Read the model definition and answer for the solid it produces. Units are mm, in the model's axes. Face numbers are marked on the shaded views. Coordinates: 2 decimals unless noted, no trailing zeros. Write each loop counter-clockwise with the first axis right and the second up, starting at its lowest first coordinate (ties: lowest second). Pieces come first, ordered by that corner, then holes. Notation, with made-up numbers: M 26.25,-16 L 78.25,-16 A16 cw 78.25,12 Z; hole C -22.75,-36 d4. An arc over 180 degrees is marked long. Write item = value, one per line.
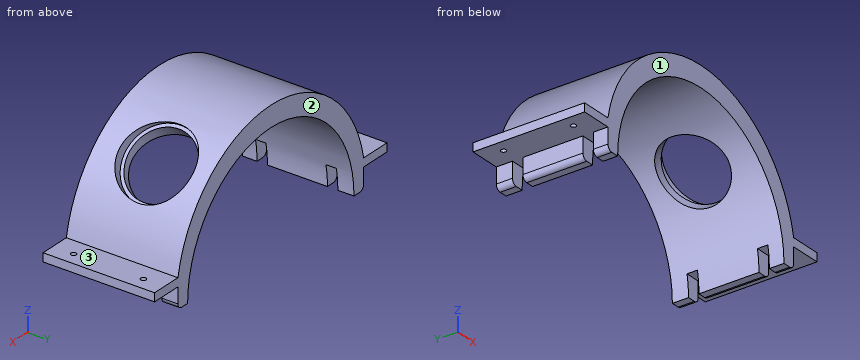
from build123d import *

# Parameters (mm, degrees)
BOSS_EXTRUDE1_DEPTH = 107
SKETCH2_R           = 2.5
CUT_EXTRUDE1_DEPTH  = 336.0337743
SKETCH3_R           = 35
CUT_EXTRUDE2_DEPTH  = 10
SKETCH4_R           = 31.778321021
CUT_EXTRUDE3_DEPTH  = 25
CUT_EXTRUDE4_REACH  = 337.034
SKETCH5_W           = 15.542799326
SKETCH5_H           = 10
SKETCH5_W_2         = 18.63674205


with BuildPart() as part:
    # Sketch1 → Boss-Extrude1 (new body)
    with BuildSketch(Plane(origin=(0, 0, 0), x_dir=(1, 0, 0), z_dir=(0, 1, 0))):
        with BuildLine():
            Line((0, 0), (0, -8))
            Line((0, -8), (30, -8))
            ThreePointArc((30, -8), (149.5, -106.759683035), (269, -8))
            Line((269, -8), (299, -8))
            Line((299, -8), (299, 0))
            Line((299, 0), (269, 0))
            Line((269, 0), (269, 15))
            ThreePointArc((269, 15), (267.535533906, 18.535533906), (264, 20))
            Line((264, 20), (256.5, 20))
            ThreePointArc((256.5, 20), (149.5, -87.000008561), (42.5, 20))
            Line((42.5, 20), (35, 20))
            ThreePointArc((35, 20), (31.464466094, 18.535533906), (30, 15))
            Line((30, 15), (30, 0))
            Line((30, 0), (0, 0))
        make_face()
    extrude(amount=BOSS_EXTRUDE1_DEPTH)

    # Sketch2 → Cut-Extrude1 (cut, through all)
    with BuildSketch(Plane(origin=(0, 0, 0), x_dir=(-1, 0, 0), z_dir=(0, 0, -1))):
        with Locations((-286.5, 87)):
            Circle(SKETCH2_R)
        with Locations((-286.5, 20)):
            Circle(SKETCH2_R)
        with Locations((-12.5, 87)):
            Circle(SKETCH2_R)
        with Locations((-12.5, 20)):
            Circle(SKETCH2_R)
    extrude(amount=-CUT_EXTRUDE1_DEPTH, mode=Mode.SUBTRACT)

    # Sketch3 → Cut-Extrude2 (cut)
    with BuildSketch(Plane(origin=(152.698962186, 0, 153.519285181), x_dir=(0.7089984938103423, 0, -0.7052099940972661), z_dir=(0.7052099940972661, 0, 0.7089984938103423))):
        with Locations((109.109605527, 56.865799068)):
            Circle(SKETCH3_R)
    extrude(amount=-CUT_EXTRUDE2_DEPTH, mode=Mode.SUBTRACT)

    # Sketch4 → Cut-Extrude3 (cut)
    with BuildSketch(Plane(origin=(145.646862245, 0, 146.429300243), x_dir=(0.7089984938103423, 0, -0.7052099940972661), z_dir=(0.7052099940972661, 0, 0.7089984938103423))):
        with Locations((109.109605527, 56.865799068)):
            Circle(SKETCH4_R)
    extrude(amount=-CUT_EXTRUDE3_DEPTH, mode=Mode.SUBTRACT)

    # Cut-Extrude4: up to this face of the body (flat: up to its plane)
    cut_extrude4_end = Plane(part.part.faces().sort_by_distance((260.25, 53.5, -20))[0])
    # Sketch5 → Cut-Extrude4 (cut, up to the picked face)
    with BuildSketch(Plane(origin=(0, 0, 0), x_dir=(-1, 0, 0), z_dir=(0, 0, -1)), mode=Mode.PRIVATE) as cut_extrude4_sk1:
        with Locations((-261.228600337, 86.535453814)):
            Rectangle(SKETCH5_W, SKETCH5_H)
    cut_extrude4_tool1 = split(extrude(cut_extrude4_sk1.sketch, amount=CUT_EXTRUDE4_REACH, mode=Mode.PRIVATE), bisect_by=cut_extrude4_end, keep=Keep.BOTH, mode=Mode.PRIVATE)
    # Sketch5 → Cut-Extrude4 (cut, up to the picked face)
    with BuildSketch(Plane(origin=(0, 0, 0), x_dir=(-1, 0, 0), z_dir=(0, 0, -1)), mode=Mode.PRIVATE) as cut_extrude4_sk2:
        with Locations((-259.681628975, 19.008712967)):
            Rectangle(SKETCH5_W_2, SKETCH5_H)
    cut_extrude4_tool2 = split(extrude(cut_extrude4_sk2.sketch, amount=CUT_EXTRUDE4_REACH, mode=Mode.PRIVATE), bisect_by=cut_extrude4_end, keep=Keep.BOTH, mode=Mode.PRIVATE)
    # Sketch5 → Cut-Extrude4 (cut, up to the picked face)
    with BuildSketch(Plane(origin=(0, 0, 0), x_dir=(-1, 0, 0), z_dir=(0, 0, -1)), mode=Mode.PRIVATE) as cut_extrude4_sk3:
        with Locations((-39.318371025, 19.008712967)):
            Rectangle(SKETCH5_W_2, SKETCH5_H)
    cut_extrude4_tool3 = split(extrude(cut_extrude4_sk3.sketch, amount=CUT_EXTRUDE4_REACH, mode=Mode.PRIVATE), bisect_by=cut_extrude4_end, keep=Keep.BOTH, mode=Mode.PRIVATE)
    # Sketch5 → Cut-Extrude4 (cut, up to the picked face)
    with BuildSketch(Plane(origin=(0, 0, 0), x_dir=(-1, 0, 0), z_dir=(0, 0, -1)), mode=Mode.PRIVATE) as cut_extrude4_sk4:
        with Locations((-37.771399663, 86.535453814)):
            Rectangle(SKETCH5_W, SKETCH5_H)
    cut_extrude4_tool4 = split(extrude(cut_extrude4_sk4.sketch, amount=CUT_EXTRUDE4_REACH, mode=Mode.PRIVATE), bisect_by=cut_extrude4_end, keep=Keep.BOTH, mode=Mode.PRIVATE)
    add(cut_extrude4_tool1.solids().sort_by(Axis((261.2286, 86.535454, 0), (0, 0, -1)))[0], mode=Mode.SUBTRACT)
    add(cut_extrude4_tool2.solids().sort_by(Axis((259.681629, 19.008713, 0), (0, 0, -1)))[0], mode=Mode.SUBTRACT)
    add(cut_extrude4_tool3.solids().sort_by(Axis((39.318371, 19.008713, 0), (0, 0, -1)))[0], mode=Mode.SUBTRACT)
    add(cut_extrude4_tool4.solids().sort_by(Axis((37.7714, 86.535454, 0), (0, 0, -1)))[0], mode=Mode.SUBTRACT)


solid = part.part
Item 1: Consider line 1 along Y through (x, z) = (286.5, 2); line 2 along Y through (x, z) = (12, 4); line 3 along Z through (x, y) = (12.5, 30). Determine where each line is inside the solid, lowest interval first. Write a range as from..to.
Worked answers:
line_1 = 0..17.5, 22.5..84.5, 89.5..107
line_2 = 0..17.55, 22.45..84.55, 89.45..107
line_3 = 0..8
Item 2: Find section D-D (x = 149.5). Determine the outline of the cut face in (y, z), and give its area (3 significant figures).
Worked answers:
outline = M 0,87 L 107,87 L 107,106.76 L 0,106.76 Z
area = 2,110 mm²
Item 3: Flat-ended cylindrical pins translate along their axes: pin 1 (10 mm diameter, centred on y = 83.5, z = 53, fed in from +X); pin 2 (6.5 mm diameter, centred on x = 12.5, y = 20, fed in from +Z); pin 3 (6 mm diameter, centred on x = 234.5, y = 38.5, fed in from -Z). Find the tip coordinate at first contact, or state that the pin passes through.
Worked answers:
pin_1 = 253.65
pin_2 = 8
pin_3 = 40.87
Item 4: For a pull along Y with two mould halves and no side action, classify the marked faces 1, 2 and 3 as released by +Y, released by -Y, zero draft, split by the parting line, or undercut.
Worked answers:
face_1 = released by -Y
face_2 = released by +Y
face_3 = zero draft
Item 5: Find section B-B (z = 26.5). Determine the outline of the cut face in (x, y).
Worked answers:
outline = M 35.09,0 L 53.13,0 L 53.13,107 L 35.09,107 Z; M 245.87,0 L 263.91,0 L 263.91,107 L 245.87,107 Z
Item 6: Find section C-C (y = 74). Determine the outline of the cut face in (x, z).
Worked answers:
outline = M 0,0 L 30,0 L 30,-15 A5 ccw 35,-20 L 42.5,-20 A107 cw 193.34,77.61 L 204.03,88.36 L 201.37,91.01 L 204.14,93.8 A121.68 ccw 30,8 L 0,8 Z; M 235.32,43.91 A107 cw 256.5,-20 L 264,-20 A5 ccw 269,-15 L 269,0 L 299,0 L 299,8 L 269,8 A121.68 ccw 250.13,53.48 L 244.64,47.96 L 241.98,50.61 Z
Item 7: Find section A-A (y = 53). Determine the outline of the cut face in (x, z).
Worked answers:
outline = M 0,0 L 30,0 L 30,-15 A5 ccw 35,-20 L 42.5,-20 A107 cw 188.58,79.61 L 200.64,91.73 L 198.34,94.02 L 200.07,95.75 A121.68 ccw 30,8 L 0,8 Z; M 238.12,39.96 A107 cw 256.5,-20 L 264,-20 A5 ccw 269,-15 L 269,0 L 299,0 L 299,8 L 269,8 A121.68 ccw 252.52,49.83 L 247.67,44.95 L 245.37,47.24 Z
